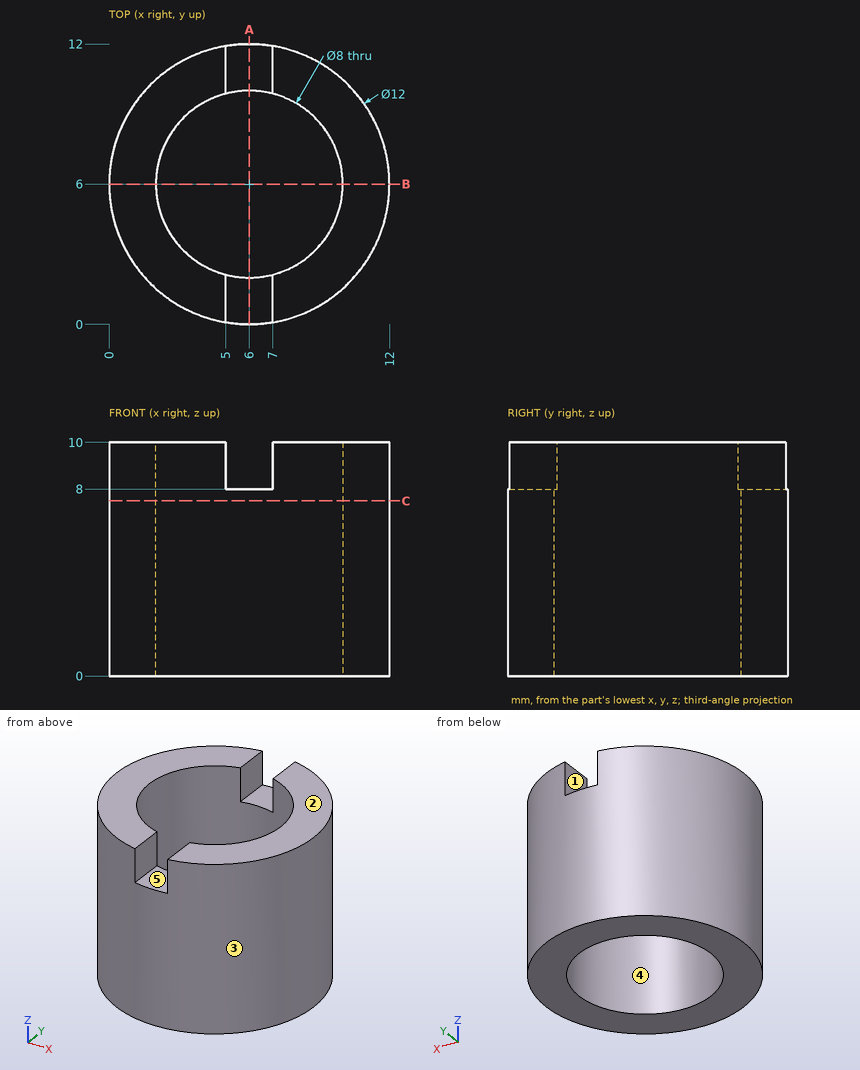
Job drawing, mm, ordinate dimensions from the low corner. One solid piece. A direction names the side the tool comes from. Give positions to 0.01 mm unless a question says otherwise; leave off trailing zeros. Loops run counter-clockwise (first coordinate to the right, second up) from the corner with the lowest first, then second, coordinate; pieces in that order, holes last. Notation, with made-up numbers: M 23.25,25.25 L 63.25,25.25 A26 ccw 63.25,57.25 Z; hole C 13.25,6 d10. An arc over 180 degrees is marked long. Return JSON: item names as keys, results as strings.
1) Pull direction Y, two halves, no side cores. Call the marked faces 3, 4 and 5: released by +Y, released by -Y, zero draft, split by the parting line, or undercut.
Calculated:
{"face 3": "split by the parting line", "face 4": "undercut", "face 5": "zero draft"}
2) Saw through at A-A, the plane x = 6. List the corners of the cut face in (y, z).
Calculated:
{"outline": "M 0,0 L 2,0 L 2,8 L 0,8 Z; M 10,0 L 12,0 L 12,8 L 10,8 Z"}
3) Saw through at C-C, the plane z = 7.5. List the corners of the cut face in (x, y).
Calculated:
{"outline": "C 6,6 d12; hole C 6,6 d8"}
4) Flat gauge pins, fed straight in: pin 1 Ø2 at (y, z) = (10.5, 9.5) entering from -X; pin 2 Ø3 at (x, z) = (10, 5.5) entering from -Y; pin 3 Ø1 at (x, y) = (7, 8.5) entering from -Z; pin 4 Ø2 at (y, z) = (10, 4.5) entering from +X. Where does each tip first touch, or does it go through?
Calculated:
{"pin 1": "stops at x = 1.13", "pin 2": "stops at y = 0.55", "pin 3": "passes through", "pin 4": "stops at x = 11.2"}
5) Drill centre lines: line 1 (Y direction, x = 6, z = 3.5); line 2 (Y direction, x = 3.75, z = 7.5); line 3 (Z direction, x = 5.5, y = 1). Where is each one in solid material? Low to high.
Calculated:
{"line 1": "y = 0 to 2, 10 to 12", "line 2": "y = 0.44 to 2.69, 9.31 to 11.56", "line 3": "z = 0 to 8"}
6) 3-axis set-ups, long thin cutter, end or side, ignore diameter. For the marked faces 1 and 2: which of +Z, -Z, +X, -X, +Y, -Y reach the whole face in a straight line?
Calculated:
{"face 1": "+Z, +Y, -Y", "face 2": "+Z, +X, -X, +Y, -Y"}
7) Saw through at B-B, the plane y = 6. List the corners of the cut face in (x, z), then the cut area to 3 significant figures.
Calculated:
{"outline": "M 0,0 L 2,0 L 2,10 L 0,10 Z; M 10,0 L 12,0 L 12,10 L 10,10 Z", "area": "40.0 mm2"}
